Solid Edge part; units mm, degrees
sketch "Sketch1" plane through (0, 0, 0) normal (0, 0, 1) x (1, 0, 0)
  arc A0 (-21, -27.4891) -> (-16.4203, -32.4714) centre (-16, -27.4891) ccw
  arc A1 (-15.1743, -33.0501) -> (-16.4203, -32.4714) centre (-16.5885, -34.4643) ccw
  line L0 (-15.1743, -33.0501) -> (21, -69.2244)
  line L1 (21, -89.8567) -> (21, -69.2244)
  arc A2 (21, -89.8567) -> (23, -91.8567) centre (23, -89.8567) ccw
  line L2 (23, -91.8567) -> (28, -91.8567)
  arc A3 (28, -91.8567) -> (30, -89.8567) centre (28, -89.8567) ccw
  line L3 (30, 89.8567) -> (30, -89.8567)
  arc A4 (28, 91.8567) -> (30, 89.8567) centre (28, 89.8567) cw
  line L4 (23, 91.8567) -> (28, 91.8567)
  arc A5 (21, 89.8567) -> (23, 91.8567) centre (23, 89.8567) cw
  line L5 (21, 89.8567) -> (21, 69.2244)
  line L6 (-15.1743, 33.0501) -> (21, 69.2244)
  arc A6 (-16.4203, 32.4714) -> (-15.1743, 33.0501) centre (-16.5885, 34.4643) ccw
  arc A7 (-16.4203, 32.4714) -> (-21, 27.4891) centre (-16, 27.4891) ccw
  line L7 (-21, 27.4891) -> (-21, -27.4891)
  circle A8 centre (-14.5, 25) radius 1.65
  circle A9 centre (-14.5, -25) radius 1.65
  arc A10 (-11.5, -18) -> (-13.5, -20) centre (-13.5, -18) cw
  line L8 (-15.5, -20) -> (-13.5, -20)
  arc A11 (-17.5, -18) -> (-15.5, -20) centre (-15.5, -18) ccw
  line L9 (-17.5, 18) -> (-17.5, -18)
  arc A12 (-15.5, 20) -> (-17.5, 18) centre (-15.5, 18) ccw
  line L10 (-13.5, 20) -> (-15.5, 20)
  arc A13 (-13.5, 20) -> (-11.5, 18) centre (-13.5, 18) cw
  line L11 (-11.5, -18) -> (-11.5, 18)
  line L12 (-5.25, -23.7446) -> (10.75, -23.7446)
  arc A14 (12.75, -25.7446) -> (10.75, -23.7446) centre (10.75, -25.7446) ccw
  line L13 (12.75, -25.7446) -> (12.75, -26.7446)
  arc A15 (10.75, -28.7446) -> (12.75, -26.7446) centre (10.75, -26.7446) ccw
  line L14 (10.75, -28.7446) -> (-5.25, -28.7446)
  arc A16 (-5.25, -28.7446) -> (-7.25, -26.7446) centre (-5.25, -26.7446) cw
  line L15 (-7.25, -26.7446) -> (-7.25, -25.7446)
  arc A17 (-7.25, -25.7446) -> (-5.25, -23.7446) centre (-5.25, -25.7446) cw
  line L16 (-5.5, -20) -> (9.25, -20)
  line L17 (9.25, 20) -> (9.25, -20)
  line L18 (-5.5, 20) -> (9.25, 20)
  arc A18 (-5.5, 20) -> (-7.5, 18) centre (-5.5, 18) ccw
  line L19 (-7.5, 18) -> (-7.5, -18)
  arc A19 (-7.5, -18) -> (-5.5, -20) centre (-5.5, -18) ccw
  line L20 (-5.25, 23.7446) -> (10.75, 23.7446)
  arc A20 (12.75, 25.7446) -> (10.75, 23.7446) centre (10.75, 25.7446) cw
  line L21 (12.75, 25.7446) -> (12.75, 26.7446)
  arc A21 (10.75, 28.7446) -> (12.75, 26.7446) centre (10.75, 26.7446) cw
  line L22 (10.75, 28.7446) -> (-5.25, 28.7446)
  arc A22 (-5.25, 28.7446) -> (-7.25, 26.7446) centre (-5.25, 26.7446) ccw
  line L23 (-7.25, 26.7446) -> (-7.25, 25.7446)
  arc A23 (-7.25, 25.7446) -> (-5.25, 23.7446) centre (-5.25, 25.7446) ccw
  arc A24 (24, 35.4891) -> (21, 32.4891) centre (21, 35.4891) cw
  line L24 (-2.4216, 32.4891) -> (21, 32.4891)
  arc A25 (-3.8358, 35.9033) -> (-2.4216, 32.4891) centre (-2.4216, 34.4891) ccw
  line L25 (-3.8358, 35.9033) -> (20.5858, 60.3249)
  arc A26 (20.5858, 60.3249) -> (24, 58.9107) centre (22, 58.9107) cw
  line L26 (24, 35.4891) -> (24, 58.9107)
extrude "Protrusion1" add sketch "Sketch1" along normal blind 5
sketch "Sketch2" plane through (0, 0, 0) normal (0, 0, 1) x (1, 0, 0)
  line L0 (-2.4216, -32.4891) -> (21, -32.4891)
  arc A0 (24, -35.4891) -> (21, -32.4891) centre (21, -35.4891) ccw
  line L1 (24, -35.4891) -> (24, -58.9107)
  arc A1 (20.5858, -60.3249) -> (24, -58.9107) centre (22, -58.9107) ccw
  line L2 (-3.8358, -35.9033) -> (20.5858, -60.3249)
  arc A2 (-3.8358, -35.9033) -> (-2.4216, -32.4891) centre (-2.4216, -34.4891) cw
extrude "ExtrudedCutout_3" cut sketch "Sketch2" along normal blind 9
sketch "Sketch3" plane through (30, 0, 2.5) normal (1, 0, 0) x (0, 1, 0)
  line L0 (-89.8567, 2.5) -> (-77.8567, 2.5)
  line L1 (-77.8567, 2.5) -> (-77.8567, 12.5)
  arc A0 (-79.8567, 14.5) -> (-77.8567, 12.5) centre (-79.8567, 12.5) cw
  line L2 (-79.8567, 14.5) -> (-87.8567, 14.5)
  arc A1 (-87.8567, 14.5) -> (-89.8567, 12.5) centre (-87.8567, 12.5) ccw
  line L3 (-89.8567, 12.5) -> (-89.8567, 2.5)
  circle A2 centre (-83.8567, 8.5) radius 2.6
  line L4 (89.8567, 2.5) -> (77.8567, 2.5)
  line L5 (77.8567, 2.5) -> (77.8567, 12.5)
  arc A3 (79.8567, 14.5) -> (77.8567, 12.5) centre (79.8567, 12.5) ccw
  line L6 (79.8567, 14.5) -> (87.8567, 14.5)
  arc A4 (87.8567, 14.5) -> (89.8567, 12.5) centre (87.8567, 12.5) cw
  line L7 (89.8567, 12.5) -> (89.8567, 2.5)
  circle A5 centre (83.8567, 8.5) radius 2.6
extrude "ExtrudedProtrusion_8" add sketch "Sketch3" against normal blind 9
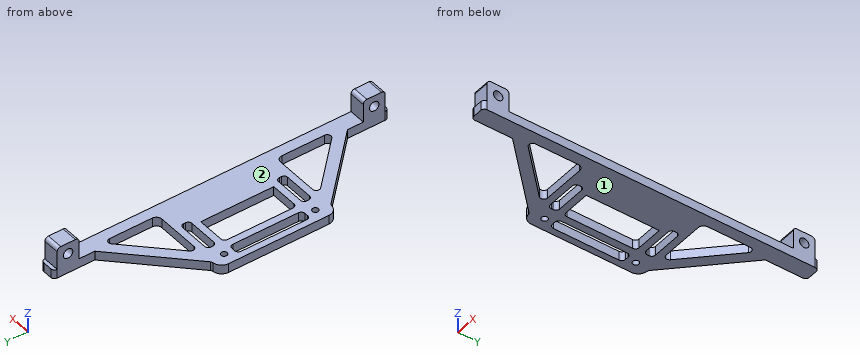
The listing builds one solid part. Answer for the finished solid, in the listing's coordinates (mm). Face numbers are marked on the shaded views. A direction names the side the tool comes from. Round coordinates to 2 decimals unless told otherwise and drop trailing zeros. Write each loop counter-clockwise with the first axis right and the second up, starting at its lowest first coordinate (ties: lowest second). Pieces come first, ordered by that corner, then holes. Notation, with made-up numbers: (9.25, -6.5) - (45.25, -6.5) arc R13 cw to (45.25, 15.5) - close; hole circle Ø7 at (42.5, 36). An arc over 180 degrees is marked (long way). Use a Markdown table: item, result. Add a question column.
1. Consider line 1 (Y direction, x = -14.5, z = 3.85); line 2 (Y direction, x = 20, z = 1.75); line 3 (Y direction, x = 23.5, z = 7.25). Determine where each line is inside the solid, lowest interval first.
2. The part is cut by section A-A (z = 11). Write down the section's boundary in (x, y).
3. Flat-ended cylindrical pins translate along their axes: P1, Ø2, axis at x = -5.5, y = 7, coming from the -Z side; P2, Ø6, axis at y = 83.86, z = 11, coming from the -X side; P3, Ø2.5, axis at x = 14, z = 3.5, coming from the -Y side; P4, Ø8, axis at x = 23, z = 9.5, coming from the +Y side. Find the tip coordinate at first contact, or state that the pin passes through.
4. The part is cut by section C-C (x = 1). Write down the section's boundary in (y, z).
5. A tool of negligible diameter and unlimited length cuts with its end or side. For the marked faces 1 and 2, from which of +Z, -Z, +X, -X, +Y, -Y can it reach the whole face along a straight path? Write none if from no direction.
6. The part is cut by section D-D (y = -45). Write down the section's boundary in (x, z).
7. The part is cut by section B-B (y = -16). Write down the section's boundary in (x, z).
Reported:
| question | item | result |
|---|---|---|
| 1 | line 1 | -33.72 to -26.65, -23.35 to -20, 20 to 23.35, 26.65 to 33.72 |
| 1 | line 2 | -68.22 to -59.74, -32.49 to 32.49, 59.74 to 68.22 |
| 1 | line 3 | -89.86 to -77.86, 77.86 to 89.86 |
| 2 | outline | (21, -89.86) - (30, -89.86) - (30, -86.46) - (21, -86.46) - close; (21, -81.26) - (30, -81.26) - (30, -77.86) - (21, -77.86) - close; (21, 77.86) - (30, 77.86) - (30, 81.26) - (21, 81.26) - close; (21, 86.46) - (30, 86.46) - (30, 89.86) - (21, 89.86) - close |
| 3 | P1 | through |
| 3 | P2 | x = 21 |
| 3 | P3 | y = -63.47 |
| 3 | P4 | y = 89.86 |
| 4 | outline | (-49.22, 0) - (-40.74, 0) - (-40.74, 5) - (-49.22, 5) - close; (-32.49, 0) - (-28.74, 0) - (-28.74, 5) - (-32.49, 5) - close; (-23.74, 0) - (-20, 0) - (-20, 5) - (-23.74, 5) - close; (20, 0) - (23.74, 0) - (23.74, 5) - (20, 5) - close; (28.74, 0) - (32.49, 0) - (32.49, 5) - (28.74, 5) - close; (40.74, 0) - (49.22, 0) - (49.22, 5) - (40.74, 5) - close |
| 5 | face 1 | -Z, +X, -X, +Y, -Y |
| 5 | face 2 | +Z, +X, -X |
| 6 | outline | (-3.22, 0) - (5.26, 0) - (5.26, 5) - (-3.22, 5) - close; (24, 0) - (30, 0) - (30, 5) - (24, 5) - close |
| 7 | outline | (-21, 0) - (-17.5, 0) - (-17.5, 5) - (-21, 5) - close; (-11.5, 0) - (-7.5, 0) - (-7.5, 5) - (-11.5, 5) - close; (9.25, 0) - (30, 0) - (30, 5) - (9.25, 5) - close |
